Build history of the part. All positions in model axes, mm. Face numbers are marked on the shaded views. A direction names the side the tool comes from. Round coordinates to 2 decimals unless told otherwise and drop trailing zeros. Loops run counter-clockwise (first coordinate to the right, second up) from the corner with the lowest first, then second, coordinate; pieces in that order, holes last. Notation, with made-up numbers: (14.25, 78) -> (46.25, 78) arc R32 ccw to (46.25, 104) -> close; hole circle Ø3 at (-12.5, 24.25). An arc over 180 degrees is marked (long way). Put each result on its own line as item: value. Start each with the question number.
Item 1: Pull direction X, two halves, no side cores. Call the marked faces 3, 4 and 5: +X half, -X half, draft (parallel to the pull), parting line (faces both ways), or undercut.
Item 2: Cut at B-B, the plane y = 0. List the corners of the cut face in (x, z), plus the area to 3 significant figures.
Item 3: Tool access for the marked faces 1 and 2: list every direction of +Z, -Z, +X, -X, +Y, -Y with a clear straight run to the whole face (end or side of a thin tool).
Item 4: Cut at A-A, the plane x = -7.5. List the corners of the cut face in (y, z).
Item 5: Drill centre lines: probe 1 along Y at (x, z) = (-3.75, 1.4); probe 2 along X at (y, z) = (-0.6, 1.2); probe 3 along X at (y, z) = (0.05, 0.5). Where is each one in solid material? Low to high. Write a range as [from, to].
Item 6: Cut at C-C, the plane z = 1.2. List the corners of the cut face in (x, y), plus the area to 3 significant figures.
```python
from build123d import *

# Parameters (mm, degrees)
SKETCH1_R           = 1
BOSS_EXTRUDE1_DEPTH = 1.5


with BuildPart() as part:
    # Sketch1 → Boss-Extrude1 (new body)
    with BuildSketch(Plane.XY):
        with BuildLine():
            Line((-10, 2), (10, 2))
            ThreePointArc((10, 2), (12, 0), (10, -2))
            Line((10, -2), (-10, -2))
            ThreePointArc((-10, -2), (-12, 0), (-10, 2))
        make_face()
        with Locations((10, 0)):
            Circle(SKETCH1_R, mode=Mode.SUBTRACT)
        with BuildLine():
            Line((-10, 1), (0, 1))
            ThreePointArc((0, 1), (1, 0), (0, -1))
            Line((0, -1), (-10, -1))
            ThreePointArc((-10, -1), (-11, 0), (-10, 1))
        make_face(mode=Mode.SUBTRACT)
    extrude(amount=BOSS_EXTRUDE1_DEPTH)


solid = part.part
```
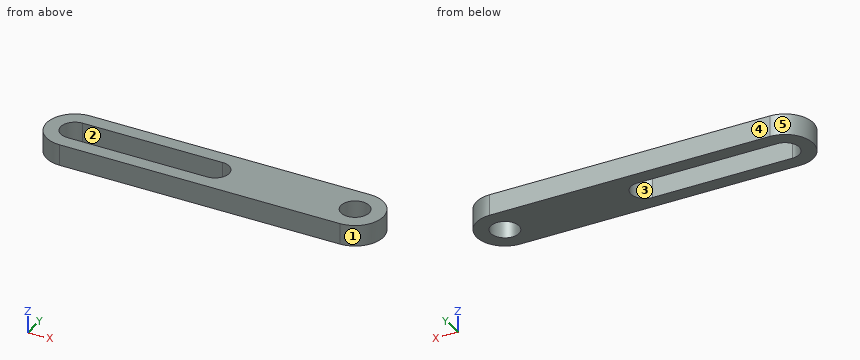
Reply:
1. face 3: undercut
1. face 4: draft
1. face 5: -X half
2. outline: (-12, 0) -> (-11, 0) -> (-11, 1.5) -> (-12, 1.5) -> close; (1, 0) -> (9, 0) -> (9, 1.5) -> (1, 1.5) -> close; (11, 0) -> (12, 0) -> (12, 1.5) -> (11, 1.5) -> close
2. area: 15.0 mm^2
3. face 1: +Z, -Z, +X
3. face 2: +Z, -Z
4. outline: (-2, 0) -> (-1, 0) -> (-1, 1.5) -> (-2, 1.5) -> close; (1, 0) -> (2, 0) -> (2, 1.5) -> (1, 1.5) -> close
5. probe 1: y = [-2, -1], [1, 2]
5. probe 2: x = [-11.91, -10.8], [0.8, 9.2], [10.8, 11.91]
5. probe 3: x = [-12, -11], [1, 9], [11, 12]
6. outline: (-10, -2) -> (10, -2) arc R2 ccw to (10, 2) -> (-10, 2) arc R2 ccw to start; hole (-10, -1) -> (0, -1) arc R1 ccw to (0, 1) -> (-10, 1) arc R1 ccw to start; hole circle Ø2 at (10, 0)
6. area: 66.3 mm^2
